For this review, take the finished solid that the model builds, in its own axes (mm). A direction names the side the tool comes from. Round coordinates to 2 decimals unless told otherwise and drop trailing zeros. Order: outer loops, then holes, each group sorted by start corner. A loop starts at its lowest first (then second) coordinate and runs counter-clockwise, first axis right, second up. Notation, with made-up numbers: M -8,25 L 28,25 A16 ccw 28,38 Z; hole C -29.5,-31.75 d7. An arc over 180 degrees is marked long. Put each result on its own line as item: value.
Autodesk Inventor part; units mm, degrees
ref_plane "YZ Plane" through (0, 0, 0) normal (1, 0, 0) x (0, 1, 0)
ref_plane "XZ Plane" through (0, 0, 0) normal (0, 1, 0) x (-1, 0, 0)
ref_plane "XY Plane" through (0, 0, 0) normal (0, 0, 1) x (1, 0, 0)
sketch "Sketch2" plane through (0, 0, 0) normal (0, 1, 0) x (-1, 0, 0)
  line L0 (15.1065, 40) -> (17.4159, 44)
  line L1 (17.4159, 44) -> (22.0347, 44)
  line L2 (22.0347, 44) -> (24.3441, 40)
  line L3 (24.3441, 40) -> (22.0347, 36)
  line L4 (22.0347, 36) -> (17.4159, 36)
  line L5 (17.4159, 36) -> (15.1065, 40)
  circle A0 centre (19.7253, 40) radius 2.55
  line L6 (-20.2747, -75) -> (-20.2747, 75)
  line L7 (0, 0) -> (41.3759, 0) construction
  line L8 (15.1065, -40) -> (17.4159, -44)
  line L9 (17.4159, -44) -> (22.0347, -44)
  line L10 (22.0347, -44) -> (24.3441, -40)
  line L11 (24.3441, -40) -> (22.0347, -36)
  line L12 (22.0347, -36) -> (17.4159, -36)
  line L13 (17.4159, -36) -> (15.1065, -40)
  circle A1 centre (19.7253, -40) radius 2.55
  line L14 (29.108, 43.6367) -> (15.0592, 55.425)
  line L15 (29.8225, 43.0372) -> (48.1619, 43.0372) construction
  line L16 (13.7736, 55.8929) -> (8.0923, 55.8929)
  line L17 (29.108, -43.6367) -> (15.0592, -55.425)
  line L18 (13.7736, -55.8929) -> (8.0923, -55.8929)
  line L19 (29.8225, 42.1046) -> (29.8225, -42.1046)
  line L20 (-20.2747, 75) -> (-6.367, 75)
  line L21 (-4.6843, 74.081) -> (6.4096, 56.812)
  arc A2 (-4.6843, 74.081) -> (-6.367, 75) centre (-6.367, 73) ccw
  arc A3 (6.4096, 56.812) -> (8.0923, 55.8929) centre (8.0923, 57.8929) ccw
  arc A4 (15.0592, 55.425) -> (13.7736, 55.8929) centre (13.7736, 53.8929) ccw
  arc A5 (29.8225, 42.1046) -> (29.108, 43.6367) centre (27.8225, 42.1046) ccw
  arc A6 (29.108, -43.6367) -> (29.8225, -42.1046) centre (27.8225, -42.1046) ccw
  arc A7 (13.7736, -55.8929) -> (15.0592, -55.425) centre (13.7736, -53.8929) ccw
  line L22 (-20.2747, -75) -> (-6.367, -75)
  line L23 (-4.6843, -74.081) -> (6.4096, -56.812)
  arc A8 (-6.367, -75) -> (-4.6843, -74.081) centre (-6.367, -73) ccw
  arc A9 (8.0923, -55.8929) -> (6.4096, -56.812) centre (8.0923, -57.8929) ccw
  point P0 (19.7253, 36)
  point P1 (19.7253, 44)
  point P2 (23.1894, 42)
  point P3 (19.7253, -36)
  point P4 (19.7253, -44)
  point P5 (23.1894, -42)
  point P6 (14.5016, 55.8929)
  point P7 (7, 55.8929)
  point P8 (29.8225, -43.0372)
  point P9 (14.5016, -55.8929)
  point P10 (7, -55.8929)
  point P11 (-5.2747, 75)
  point P12 (-5.2747, -75)
  dimension "d18" = 8
  dimension "d19" = 5.1
  dimension "d60" = 150
  dimension "d62" = 40
  dimension "d63" = 40
  dimension "d64" = 20
  dimension "d65" = 140
  dimension "d66" = 75
  dimension "d67" = 15
  dimension "d68" = 2
  dimension "d69" = 15
  dimension "d70" = 2
extrude "Extrusion11" add sketch "Sketch2" along normal blind 5 contours L6 L20 A2 L21 A3 L16 A4 L14 A5 L19 A6 L17 A7 L18 A9 L23 A8 L22
extrude "Extrusion12" add sketch "Sketch2" along normal blind 3 contours L0 L1 L2 L3 L4 L5 | L13 L12 L11 L10 L9 L8
sketch "Sketch5" plane through (0, 5, 0) normal (0, 1, 0) x (1, 0, 0)
  line L0 (6.367, -75) -> (20.2747, -75)
  line L1 (20.2747, -75) -> (20.2747, 75)
  line L2 (6.367, -75) -> (20.2747, -75)
  line L3 (20.2747, -75) -> (20.2747, 75)
  line L4 (20.2747, 75) -> (6.367, 75)
  line L5 (6.367, 75) -> (6.367, -75)
  point P0 (0, 0)
extrude "Extrusion13" add sketch "Sketch5" along normal blind 80
fillet "Fillet1" radius 5 6 edges at (6.367, 45, 75) (20.2747, 42.5, 75) (6.367, 85, 0) (20.2747, 85, 0) (6.367, 45, -75) (20.2747, 42.5, -75)
sketch "Sketch6" plane through (6.367, 5, -70) normal (-1, 0, 0) x (0, 0, 1)
  line L0 (0, 0) -> (0, 75)
  line L1 (140, 75) -> (140, 0) construction
  line L2 (140, 0) -> (140, 75)
  line L3 (145, 80) -> (145, -5)
  line L4 (0, 75) -> (140, 75)
  line L5 (115, 75) -> (115, 0) construction
  line L6 (85, 75) -> (85, 0) construction
  line L7 (50, 75) -> (50, 0) construction
  line L8 (15, 75) -> (15, 0) construction
  line L9 (140, -5) -> (140, 75)
  circle A0 centre (115, 55) radius 3
  circle A1 centre (85, 55) radius 2.5
  circle A2 centre (50, 55) radius 2.5
  circle A3 centre (15, 55) radius 3.075
  circle A4 centre (115, 55) radius 5.7
  circle A5 centre (85, 55) radius 5
  circle A6 centre (115, 20) radius 2.5
  circle A7 centre (85, 20) radius 5.1
  circle A8 centre (50, 20) radius 1.55
  circle A9 centre (15, 20) radius 4.05
  line L10 (140, 20) -> (0, 20) construction
  line L11 (140, 55) -> (0, 55) construction
  point P0 (70, -5)
  dimension "d79" = 75
  dimension "d82" = 25
  dimension "d83" = 30
  dimension "d84" = 35
  dimension "d85" = 35
  dimension "d86" = 20
  dimension "d87" = 6
  dimension "d88" = 11.4
  dimension "d89" = 5
  dimension "d90" = 10
  dimension "d91" = 5
  dimension "d92" = 6.15
  dimension "d93" = 20
  dimension "d94" = 5
  dimension "d95" = 10.2
  dimension "d96" = 3.1
  dimension "d97" = 8.1
extrude "Extrusion14" cut sketch "Sketch6" against normal through all contours A0 | A1 | A2 | A3 | A6 | A7 | A8 | A9
extrude "Extrusion15" cut sketch "Sketch6" against normal blind 6 contours A4
extrude "Extrusion16" cut sketch "Sketch6" against normal blind 3.75 contours A5
properties part number "soporte_destornillador"
(1) Insertion check: pin 1 Ø1 at (x, z) = (-7, 15) entering from -Y; pin 2 Ø8 at (y, z) = (61, 15.5) entering from -X; pin 3 Ø1.5 at (x, y) = (-11.5, 3) entering from +Z; pin 4 Ø3 at (x, z) = (-24, 31) entering from +Y. Each pin has a flat end and moves straight along its axis. Give the tip position at first contact, or say it passes through.
A:
pin 1: stops at y = 0
pin 2: stops at x = 6.37
pin 3: stops at z = 55.89
pin 4: stops at y = 5
(2) To check wall thickness, follow L1, parallel to Y at x = 13.5, z = -20; L2, parallel to Y at x = 16.5, z = -55 (3 decimals); L3, parallel to X at y = 16.5, z = 44.5. State the ranges of each line that lie inside material, in increasing order.
A:
L1: y = 0 to 23.45, 26.55 to 57.5, 62.5 to 85
L2: y = 0 to 20.95, 29.05 to 56.925, 63.075 to 84.848
L3: x = 6.37 to 20.27
(3) Add section C-C on z = -20. Give the boundary of the cut face in (x, y), then the cut area to 3 significant figures.
A:
outline: M -29.82,0 L 20.27,0 L 20.27,23.45 L 6.37,23.45 L 6.37,5 L -29.82,5 Z; M 6.37,26.55 L 20.27,26.55 L 20.27,57.5 L 6.37,57.5 Z; M 6.37,62.5 L 20.27,62.5 L 20.27,80 A5 ccw 15.27,85 L 11.37,85 A5 ccw 6.37,80 Z
area: 1,240 mm2
(4) Add section B-B on y = 25. Give the boundary of the cut face in (x, z).
A:
outline: M 6.37,-70 A5 ccw 11.37,-75 L 15.27,-75 A5 ccw 20.27,-70 L 20.27,-59.05 L 6.37,-59.05 Z; M 6.37,-50.95 L 20.27,-50.95 L 20.27,-21.55 L 6.37,-21.55 Z; M 6.37,-18.45 L 20.27,-18.45 L 20.27,9.9 L 6.37,9.9 Z; M 6.37,20.1 L 20.27,20.1 L 20.27,42.5 L 6.37,42.5 Z; M 6.37,47.5 L 20.27,47.5 L 20.27,70 A5 ccw 15.27,75 L 11.37,75 A5 ccw 6.37,70 Z
(5) For faces 1 (the face through (9.325, 54.436, 43.764)), 2 (the face through (7.793, 45.56, 73.496)), 3 (the face through (-11, 2, 55.893)), 4 (the face through (7.9, 45.6, -73.6)), list the 3-axis set-ups (+Z, -Z, +X, -X, +Y, -Y) from which the entire face can be reached by the end or side of a thin tool; tool diameter is ignored.
A:
face 1: -X
face 2: +Z, -X, +Y
face 3: +Z, -X, +Y, -Y
face 4: -Z, -X, +Y
(6) Add section D-D on y = 60. State how many separate pieces and enclosed holes the cut face has, then the cut area to 3 significant figures.
A:
separate pieces: 5
enclosed holes: 0
area: 1,710 mm2
(7) Add section A-A on z = 15. Give the boundary of the cut face in (x, y), then the cut area to 3 significant figures.
A:
outline: M -29.82,0 L 20.27,0 L 20.27,19.9 L 6.37,19.9 L 6.37,5 L -29.82,5 Z; M 6.37,30.1 L 20.27,30.1 L 20.27,57.5 L 10.12,57.5 L 10.12,55 L 6.37,55 Z; M 6.37,65 L 10.12,65 L 10.12,62.5 L 20.27,62.5 L 20.27,80 A5 ccw 15.27,85 L 11.37,85 A5 ccw 6.37,80 Z
area: 1,120 mm2
